Drawing for the job (mm, zero at the part's lowest x, y, z). Round coordinates to 2 decimals unless told otherwise and drop trailing zeros. Write each loop counter-clockwise with the first axis right and the second up, starting at its lowest first coordinate (ties: lowest second). Pieces come first, ordered by that corner, then holes. Notation, with made-up numbers: (-15.5, 43) -> (26.5, 43) arc R24 cw to (26.5, 79) -> close; hole circle Ø7 at (28.25, 16.5). An arc over 180 degrees is marked (long way). One line per question, with ' | ' between items.
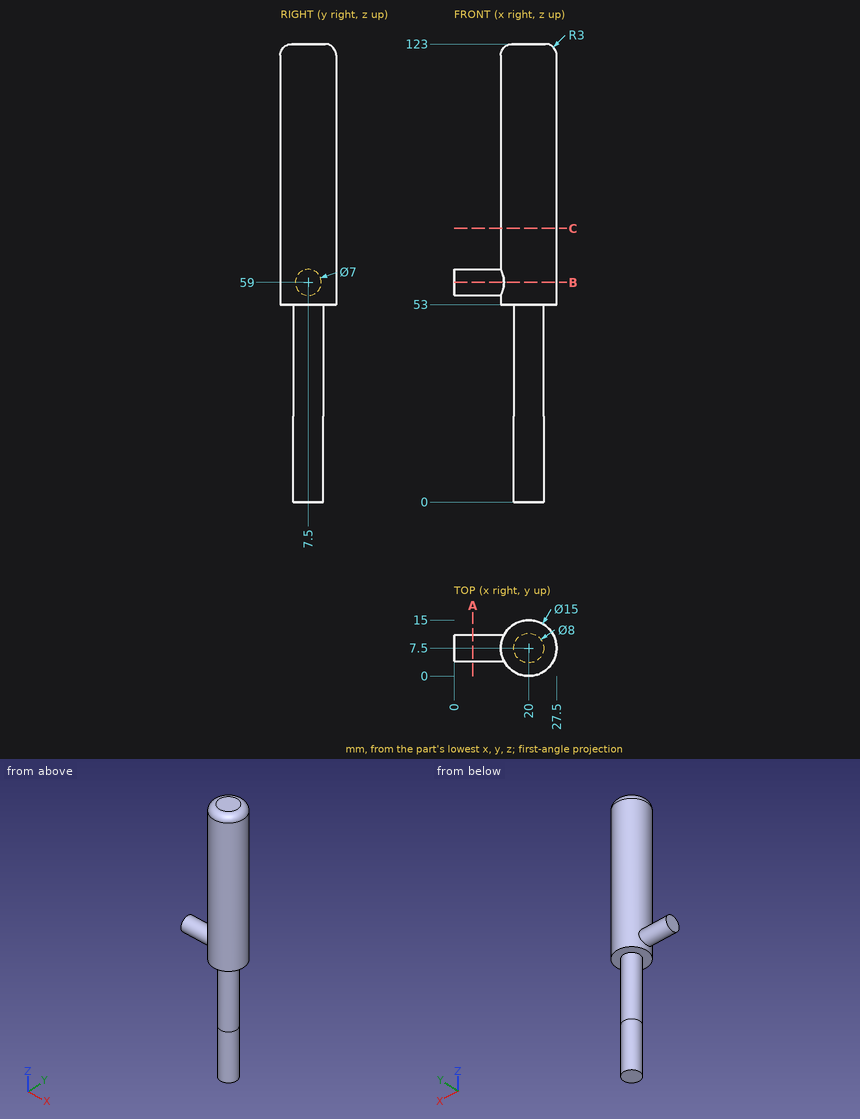
(1) Slice it at B-B (z = 59). Write the cut outline in (x, y), then the cut area to 3 significant figures.
Calculated:
outline: (0, 4) -> (13.37, 4) arc R7.5 ccw (long way) to (13.37, 11) -> (0, 11) -> close | area: 266 mm2
(2) Wall check: line 1 (Z direction, x = 20.5, y = 12.25); line 2 (Y direction, x = 14, z = 82); line 3 (Y direction, x = 21.5, z = 13). Give the ranges that are in metal, low to high. Write a range as from..to.
Calculated:
line 1: 53..122.99 | line 2: 3..12 | line 3: 3.79..11.21
(3) Drop flat-ended pins along their axis: pin 1 (1 mm diameter, centred on y = 6.5, z = 99.5, fed in from -X); pin 2 (1.5 mm diameter, centred on x = 7.5, y = 7, fed in from -Z); pin 3 (1.5 mm diameter, centred on y = 6, z = 24.5, fed in from +X). Give the stop position or say it passes through.
Calculated:
pin 1: x = 12.52 | pin 2: z = 55.5 | pin 3: x = 23.93
(4) Slice it at A-A (x = 5). Write the cut outline in (y, z), then the cut area to 3 significant figures.
Calculated:
outline: circle Ø7 at (7.5, 59) | area: 38.5 mm2
(5) Slice it at C-C (z = 73.5). Write the cut outline in (x, y).
Calculated:
outline: circle Ø15 at (20, 7.5)
